The listing builds one solid part. Answer for the finished solid, in the listing's coordinates (mm). A direction names the side the tool comes from. Round coordinates to 2 decimals unless told otherwise and drop trailing zeros. Loops run counter-clockwise (first coordinate to the right, second up) from the corner with the lowest first, then second, coordinate; pieces in that order, holes last. Notation, with made-up numbers: (69, 41.5) -> (97, 41.5) arc R23 cw to (97, 60.5) -> close; hole circle Ø4 at (55.5, -29). An arc over 180 degrees is marked (long way). Use a Markdown table: item, result. Add a question column.
Q1. Which of the six approach directions +Z, -Z, +X, -X, +Y, -Y give full straight-line access (tool end or side, diameter ignored) to faces 5 (the flat face through (72, 0, 3)), 6 (the flat face through (72, 15, 3)), 7 (the cylindrical face through (90, 8, 10)), 8 (the flat face through (-44, 30, 10))?
Q2. Section C-C on y = -8.5 is taken. Give the vertices of the cut face in (x, z).
Q3. Section B-B on x = 0 is taken. Give the vertices of the cut face in (y, z), then the cut area to 3 significant figures.
Q4. Given pin 1 Ø10 at (y, z) = (-34, 17) entering from -X; pin 2 Ø8 at (x, z) = (11.5, 4) entering from +Y; pin 3 Ø12 at (x, z) = (-34.5, 9) entering from -Y, each flat-ended and moving along its own axis, determine where each tip first touches the part or whether it passes through.
Q5. Section D-D on y = -30 is taken. Give the vertices of the cut face in (x, z).
Q6. Consider line 1 (Y direction, x = 0, z = 14.25); line 2 (X direction, y = -4.5, z = 6.5); line 3 (Y direction, x = -20, z = 17). Determine where each line is inside the solid, lowest interval first.
Q7. Section A-A on z = 10 is taken. Give the vertices of the cut face in (x, y), then the cut area to 3 significant figures.
Q8. For a pull along Z with two mould halves and no side action, classify faces 1 (the flat face through (70, 8, 5)), 2 (the flat face through (-70, 24, 10)), 3 (the flat face through (70, 8, 15)), 4 (the flat face through (-23, 13, 20)) as released by +Z, released by -Z, zero draft, split by the parting line, or undercut.
from build123d import *

# Parameters (mm, degrees)
SKETCH1_R           = 25
BOSS_EXTRUDE1_DEPTH = 20
CUT_EXTRUDE1_DEPTH  = 61


with BuildPart() as part:
    # Sketch1 → Boss-Extrude1 (new body)
    with BuildSketch(Plane.XY):
        with BuildLine():
            Line((-70, 0), (-28.928571429, -34.469374162))
            ThreePointArc((-28.928571429, -34.469374162), (19.015970731, -40.784713523), (45, 0))
            Line((45, 0), (100, 0))
            Line((100, 0), (100, 15))
            Line((100, 15), (42.426406871, 15))
            ThreePointArc((42.426406871, 15), (8.717082451, 44.14762138), (-33.541019662, 30))
            Line((-33.541019662, 30), (-55, 30))
            Line((-55, 30), (-55, 62))
            Line((-55, 62), (-70, 47))
            Line((-70, 47), (-70, 0))
        make_face()
        Circle(SKETCH1_R, mode=Mode.SUBTRACT)
    extrude(amount=BOSS_EXTRUDE1_DEPTH)

    # Sketch2 → Cut-Extrude1 (cut, through all)
    with BuildSketch(Plane(origin=(0, 15, 0), x_dir=(1, 0, 0), z_dir=(0, 1, 0))):
        with BuildLine():
            Line((55, -15), (85, -15))
            ThreePointArc((85, -15), (90, -10), (85, -5))
            Line((85, -5), (55, -5))
            ThreePointArc((55, -5), (50, -10), (55, -15))
        make_face()
    extrude(amount=-CUT_EXTRUDE1_DEPTH, mode=Mode.SUBTRACT)


solid = part.part
Checked values:
| question | item | result |
|---|---|---|
| 1 | face 5 | +Z, -Z, +X, -Y |
| 1 | face 6 | +Z, -Z, +X, +Y |
| 1 | face 7 | +Y, -Y |
| 1 | face 8 | +Z, -Z, +Y |
| 2 | outline | (-59.87, 0) -> (-23.51, 0) -> (-23.51, 20) -> (-59.87, 20) -> close; (23.51, 0) -> (44.19, 0) -> (44.19, 20) -> (23.51, 20) -> close |
| 3 | outline | (-45, 0) -> (-25, 0) -> (-25, 20) -> (-45, 20) -> close; (25, 0) -> (45, 0) -> (45, 20) -> (25, 20) -> close |
| 3 | area | 800 mm2 |
| 4 | pin 1 | stops at x = -35.45 |
| 4 | pin 2 | stops at y = 44.37 |
| 4 | pin 3 | stops at y = -34.82 |
| 5 | outline | (-34.25, 0) -> (33.54, 0) -> (33.54, 20) -> (-34.25, 20) -> close |
| 6 | line 1 | y = -45 to -25, 25 to 45 |
| 6 | line 2 | x = -64.64 to -24.59, 24.59 to 44.77 |
| 6 | line 3 | y = -40.31 to -15, 15 to 40.31 |
| 7 | outline | (-70, 0) -> (-28.93, -34.47) arc R45 ccw to (45, 0) -> (50, 0) -> (50, 15) -> (42.43, 15) arc R45 ccw to (-33.54, 30) -> (-55, 30) -> (-55, 62) -> (-70, 47) -> close; (90, 0) -> (100, 0) -> (100, 15) -> (90, 15) -> close; hole circle Ø50 at (0, 0) |
| 7 | area | 6,180 mm2 |
| 8 | face 1 | undercut |
| 8 | face 2 | zero draft |
| 8 | face 3 | undercut |
| 8 | face 4 | released by +Z |
